The model under review builds one solid part; all positions refer to its coordinate system, in mm. Coordinates: 2 decimals unless noted, no trailing zeros. Write each loop counter-clockwise with the first axis right and the second up, starting at its lowest first coordinate (ties: lowest second). Pieces come first, ordered by that corner, then holes. Notation, with made-up numbers: (47.5, 12) - (52.5, 12) arc R24 cw to (52.5, 51) - close; hole circle Ø10 at (15.5, 53). An arc over 180 degrees is marked (long way). Answer as CSV lines item,"result". Start each with the question number.
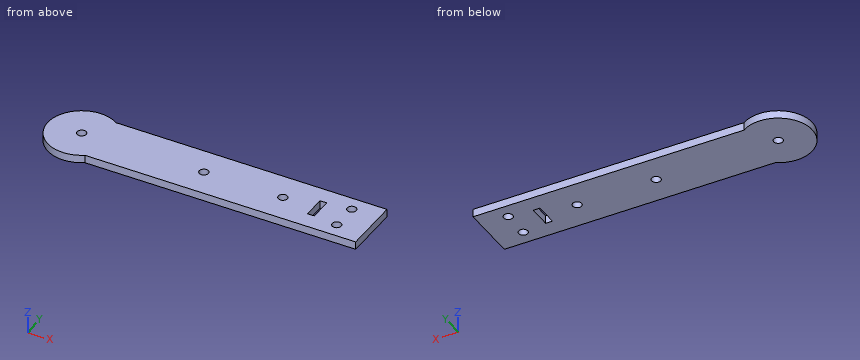
```python
from build123d import *

# Parameters (mm, degrees)
CROQUIS1_R              = 2
CROQUIS1_W              = 3
CROQUIS1_H              = 10
SALIENTE_EXTRUIR2_DEPTH = 3.5


with BuildPart() as part:
    # Croquis1 → Saliente-Extruir2 (new body)
    with BuildSketch(Plane.XY):
        with BuildLine():
            Line((34.902189702, 12.5), (34.902189702, -12.5))
            Line((34.902189702, -12.5), (-85.097810298, -12.5))
            ThreePointArc((-85.097810298, -12.5), (-108.389372273, 0), (-85.097810298, 12.5))
            Line((-85.097810298, 12.5), (34.902189702, 12.5))
        make_face()
        with Locations((-93.389372273, 0)):
            Circle(CROQUIS1_R, mode=Mode.SUBTRACT)
        with Locations((22.902189702, 6)):
            Circle(CROQUIS1_R, mode=Mode.SUBTRACT)
        with Locations((22.902189702, -6)):
            Circle(CROQUIS1_R, mode=Mode.SUBTRACT)
        with Locations((-39.291561976, 0)):
            Circle(CROQUIS1_R, mode=Mode.SUBTRACT)
        with Locations((-4.291561976, 0)):
            Circle(CROQUIS1_R, mode=Mode.SUBTRACT)
        with Locations((10.902189702, 0)):
            Rectangle(CROQUIS1_W, CROQUIS1_H, mode=Mode.SUBTRACT)
    extrude(amount=SALIENTE_EXTRUIR2_DEPTH)


solid = part.part
```
(1) Add section C-C on x = -33. Give the boundary of the cut face in (y, z), then the cut area to 3 significant figures.
(2) Add section B-B on z = 2.1. Give the boundary of the cut face in (x, y), then the cut area to 3 significant figures.
(3) Add section A-A on y = 0. Give the boundary of the cut face in (x, z), then the cut area to 3 significant figures.
(4) Add section D-D on y = 9.5. Give the boundary of the cut face in (x, z), then the cut area to 3 significant figures.
(5) Wall thickness on line 1 (Y direction, x = 7, z = 1.8); line 2 (Y direction, x = -4, z = 3.1); line 3 (X direction, y = 6.25, z = 0.9): over which ranges is each line inside the solid? List them lowest first.
(6) For pin 1 (1.5 mm diameter, centred on x = 6, z = 0.5, fed in from +Y); pin 2 (0.9 mm diameter, centred on x = 10, z = 2, fed in from -Y); pin 3 (1 mm diameter, centred on y = -9.5, z = 2, fed in from -X); pin 4 (2.5 mm diameter, centred on x = 22.9, y = -6, fed in from -Z), all flat-tipped, find the tip position at first contact; note any pin that passes through.
Reported:
1,outline,"(-12.5, 0) - (12.5, 0) - (12.5, 3.5) - (-12.5, 3.5) - close"
1,area,"87.5 mm²"
2,outline,"(-85.1, -12.5) - (34.9, -12.5) - (34.9, 12.5) - (-85.1, 12.5) arc R15 ccw (long way) to start; hole circle Ø4 at (-93.39, 0); hole circle Ø4 at (-39.29, 0); hole circle Ø4 at (-4.29, 0); hole (9.4, -5) - (12.4, -5) - (12.4, 5) - (9.4, 5) - close; hole circle Ø4 at (22.9, -6); hole circle Ø4 at (22.9, 6)"
2,area,"3,500 mm²"
3,outline,"(-108.39, 0) - (-95.39, 0) - (-95.39, 3.5) - (-108.39, 3.5) - close; (-91.39, 0) - (-41.29, 0) - (-41.29, 3.5) - (-91.39, 3.5) - close; (-37.29, 0) - (-6.29, 0) - (-6.29, 3.5) - (-37.29, 3.5) - close; (-2.29, 0) - (9.4, 0) - (9.4, 3.5) - (-2.29, 3.5) - close; (12.4, 0) - (34.9, 0) - (34.9, 3.5) - (12.4, 3.5) - close"
3,area,"449 mm²"
4,outline,"(-105, 0) - (34.9, 0) - (34.9, 3.5) - (-105, 3.5) - close"
4,area,"490 mm²"
5,line 1,"-12.5 to 12.5"
5,line 2,"-12.5 to -1.98, 1.98 to 12.5"
5,line 3,"-107.03 to 20.92, 24.89 to 34.9"
6,pin 1,"y = 12.5"
6,pin 2,"y = -12.5"
6,pin 3,"x = -105.39"
6,pin 4,"through"
